Could you check a few things on this model? Use its own coordinates, in mm. Face numbers are marked on the shaded views. A direction names the side the tool comes from. Give positions to 0.01 mm unless a question says otherwise; leave off trailing zeros. Loops run counter-clockwise (first coordinate to the right, second up) from the corner with the lowest first, then second, coordinate; pieces in that order, holes last. Notation, with made-up numbers: (-2, 33) - (15, 33) arc R15 cw to (15, 46) - close; hole circle Ø7 at (50, 31). An arc over 180 degrees is marked (long way). Write each question's results on one line, items separated by ' | '. Start each with the question number.
(1) Suppose I cut it at A-A (x = -11.25). Please give me the cut outline in (y, z), and give its area (3 significant figures).
(2) Suppose I cut it at D-D (z = 28). Please give me the cut outline in (x, y), and give its area (3 significant figures).
(3) Suppose I cut it at C-C (x = -8). Please give me the cut outline in (y, z).
(4) On a 3-axis mill with a long thin cutter (end or side, diameter ignored), from which of +Z, -Z, +X, -X, +Y, -Y can I reach the whole of each face in a straight line? I mean the marked faces 1 and 2. Say none if no direction works.
(5) I need wall thicknesses on line 1 (Y direction, x = -1, z = 16); line 2 (X direction, y = -4.5, z = 15.5); line 3 (X direction, y = -8.9, z = 5). Which ranges of each line are inside material? Lowest first, please.
(6) Suppose I cut it at B-B (z = 5). Please give me the cut outline in (x, y), and give its area (3 significant figures).
(7) For pin 1 (3 mm diameter, centred on x = -7.57, z = 5, fed in from +Y); pin 2 (2 mm diameter, centred on y = -4, z = 5, fed in from -X), each with a flat end and sliding along its axis, tell me the tip position at first contact or that it passes through.
from build123d import *

# Parameters (mm, degrees)
AUFSATZ_LINEAR_AUSTRAGEN1_DEPTH = 40
SCHNITT_LINEAR_AUSTRAGEN1_REACH = 49.036
SKIZZE2_R                       = 2.6


with BuildPart() as part:
    # Skizze1 → Aufsatz-Linear austragen1 (new body)
    with BuildSketch(Plane(origin=(0, 0, 0), x_dir=(0, 1, 0), z_dir=(0, 0, 1))):
        with BuildLine():
            Line((5.5, -5.425677432), (-5.5, -5.425677432))
            ThreePointArc((-5.5, -5.425677432), (-8.681980515, -4.107657947), (-10, -0.925677432))
            Line((-10, -0.925677432), (-10, 14.574322568))
            Line((-10, 14.574322568), (-8.5, 14.574322568))
            Line((-8.5, 14.574322568), (-8.5, -0.925677432))
            ThreePointArc((-8.5, -0.925677432), (-7.621320344, -3.046997775), (-5.5, -3.925677432))
            Line((-5.5, -3.925677432), (5.5, -3.925677432))
            ThreePointArc((5.5, -3.925677432), (7.621320344, -3.046997775), (8.5, -0.925677432))
            Line((8.5, -0.925677432), (8.5, 14.574322568))
            Line((8.5, 14.574322568), (10, 14.574322568))
            Line((10, 14.574322568), (10, -0.925677432))
            ThreePointArc((10, -0.925677432), (8.681980515, -4.107657947), (5.5, -5.425677432))
        make_face()
    extrude(amount=AUFSATZ_LINEAR_AUSTRAGEN1_DEPTH)

    # Schnitt-Linear austragen1: up to this face of the body (flat: up to its plane)
    schnitt_linear_austragen1_end = Plane(part.part.faces().sort_by_distance((-6.824322568, 10, 20))[0])
    # Skizze2 → Schnitt-Linear austragen1 (cut, up to the picked face)
    with BuildSketch(Plane.XZ.offset(10), mode=Mode.PRIVATE) as schnitt_linear_austragen1_sk1:
        with Locations(Location((-7.574322568, 35, 0), (0, 0, 270))):
            Circle(SKIZZE2_R)
    schnitt_linear_austragen1_tool1 = split(extrude(schnitt_linear_austragen1_sk1.sketch, amount=-SCHNITT_LINEAR_AUSTRAGEN1_REACH, mode=Mode.PRIVATE), bisect_by=schnitt_linear_austragen1_end, keep=Keep.BOTH, mode=Mode.PRIVATE)
    # Skizze2 → Schnitt-Linear austragen1 (cut, up to the picked face)
    with BuildSketch(Plane.XZ.offset(10), mode=Mode.PRIVATE) as schnitt_linear_austragen1_sk2:
        with Locations(Location((-7.574322568, 5, 0), (0, 0, 270))):
            Circle(SKIZZE2_R)
    schnitt_linear_austragen1_tool2 = split(extrude(schnitt_linear_austragen1_sk2.sketch, amount=-SCHNITT_LINEAR_AUSTRAGEN1_REACH, mode=Mode.PRIVATE), bisect_by=schnitt_linear_austragen1_end, keep=Keep.BOTH, mode=Mode.PRIVATE)
    add(schnitt_linear_austragen1_tool1.solids().sort_by(Axis((-7.574323, -10, 35), (0, 1, 0)))[0], mode=Mode.SUBTRACT)
    add(schnitt_linear_austragen1_tool2.solids().sort_by(Axis((-7.574323, -10, 5), (0, 1, 0)))[0], mode=Mode.SUBTRACT)


solid = part.part
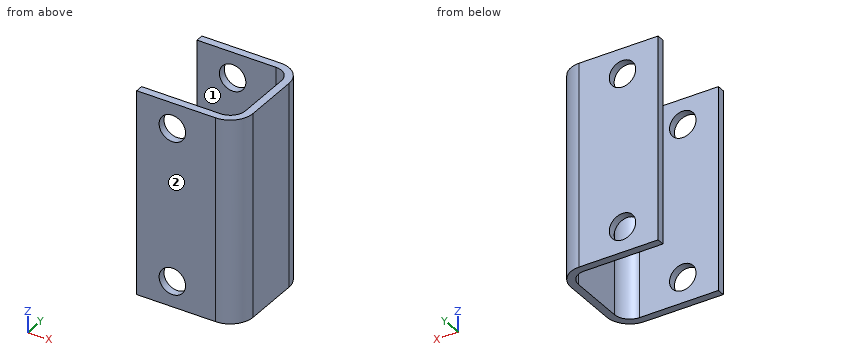
Output values:
1) outline: (-10, 0) - (-8.5, 0) - (-8.5, 40) - (-10, 40) - close; (8.5, 0) - (10, 0) - (10, 40) - (8.5, 40) - close | area: 120 mm2
2) outline: (-14.57, -10) - (0.93, -10) arc R4.5 ccw to (5.43, -5.5) - (5.43, 5.5) arc R4.5 ccw to (0.93, 10) - (-14.57, 10) - (-14.57, 8.5) - (0.93, 8.5) arc R3 cw to (3.93, 5.5) - (3.93, -5.5) arc R3 cw to (0.93, -8.5) - (-14.57, -8.5) - close | area: 80.7 mm2
3) outline: (-10, 0) - (-8.5, 0) - (-8.5, 2.44) - (-10, 2.44) - close; (-10, 7.56) - (-8.5, 7.56) - (-8.5, 32.44) - (-10, 32.44) - close; (-10, 37.56) - (-8.5, 37.56) - (-8.5, 40) - (-10, 40) - close; (8.5, 0) - (10, 0) - (10, 2.44) - (8.5, 2.44) - close; (8.5, 7.56) - (10, 7.56) - (10, 32.44) - (8.5, 32.44) - close; (8.5, 37.56) - (10, 37.56) - (10, 40) - (8.5, 40) - close
4) face 1: +Z, -Z, -X | face 2: +Z, -Z, +X, -X, -Y
5) line 1: -10 to -8.5, 8.5 to 10 | line 2: 3.93 to 5.43 | line 3: -14.57 to -10.17, -4.97 to 3.87
6) outline: (-14.57, -10) - (-10.17, -10) - (-10.17, -8.5) - (-14.57, -8.5) - close; (-14.57, 8.5) - (-10.17, 8.5) - (-10.17, 10) - (-14.57, 10) - close; (-4.97, -10) - (0.93, -10) arc R4.5 ccw to (5.43, -5.5) - (5.43, 5.5) arc R4.5 ccw to (0.93, 10) - (-4.97, 10) - (-4.97, 8.5) - (0.93, 8.5) arc R3 cw to (3.93, 5.5) - (3.93, -5.5) arc R3 cw to (0.93, -8.5) - (-4.97, -8.5) - close | area: 65.1 mm2
7) pin 1: through | pin 2: x = 3.93
